Source: CAD feature listing. Evaluate the final solid. Frame: model axes, mm. A direction names the side the tool comes from. Round coordinates to 2 decimals unless told otherwise and drop trailing zeros. Write each loop counter-clockwise with the first axis right and the second up, starting at its lowest first coordinate (ties: lowest second). Pieces come first, ordered by that corner, then holes. Notation, with made-up numbers: (8, 58.5) -> (17, 58.5) arc R16 ccw to (17, 70.5) -> close; hole circle Ø1 at (-8, -17). An arc over 180 degrees is marked (long way). Return JSON: item names as keys, results as strings. Group by question number.
Autodesk Fusion 360 part; units mm, degrees
sketch "Sketch1" plane through (0, 0, 0) normal (0, 0, 1) x (1, 0, 0)
  circle A0 centre (0, 0) radius 12
  dimension "d1" = 24
extrude "Extrude1" add sketch "Sketch1" along normal blind 16.75 makes body 1
sketch "Sketch2" plane through (0, 0, 0) normal (0, 0, 1) x (1, 0, 0)
  circle A0 centre (0, 0) radius 19.75
  dimension "d4" = 39.5
extrude "Extrude2" add sketch "Sketch2" against normal blind 13 bodies 1
sketch "Sketch3" plane through (0, 0, 0) normal (0, 1, 0) x (1, 0, 0)
  line L0 (0, 0) -> (0, -4.94)
  dimension "d7" = 4.94
sketch "Sketch4" plane through (0, 0, 16.75) normal (0, 0, 1) x (-1, 0, 0)
  circle A0 centre (0, 0) radius 12
sketch "Sketch5" plane through (0, 0, 0) normal (0, 1, 0) x (1, 0, 0)
sketch "Sketch6" plane through (0, 0, 0) normal (0, 0, 1) x (1, 0, 0)
  circle A0 centre (0, 0) radius 16
  dimension "d9" = 32
extrude "Extrude3" add sketch "Sketch6" along normal blind 3 separate body makes body 2
move_body "Move1" bodies 2 to x (1, 0, 0) y (0, 1, 0) z (0, 0, 1) at (0, 0, 4.94)
sketch "Sketch7" plane through (0, 0, 7.94) normal (0, 0, 1) x (-1, 0, 0)
  circle A0 centre (0, 0) radius 16
  line L0 (0, 0) -> (13, 16)
  line L1 (0, -2.5) -> (0, -20)
  line L2 (0, 0) -> (-13, 16)
  line L3 (-20, 0) -> (-2.5, 0)
  line L4 (0, 0) -> (13, -16)
  line L5 (0, 0) -> (-13, -16)
  line L6 (-13, 16) -> (-22, 6)
  line L7 (-22, 6) -> (-13, -16)
  line L8 (13, 16) -> (27, 0)
  line L9 (27, 0) -> (13, -16)
extrude "Extrude4" cut sketch "Sketch7" against normal blind 4 contours A0 L0 L4 | A0 L0 L4 L8 L9 | A0 L2 L5 | A0 L2 L3 L6 L7 | A0 L3 L5 L7 bodies 2
sketch "Sketch8" plane through (0, 0, 16.75) normal (0, 0, 1) x (-1, 0, 0)
  circle A0 centre (0, 0) radius 7
  dimension "d14" = 14
extrude "Extrude5" cut sketch "Sketch8" against normal blind 33 bodies 1 2 makes body 3 at (-4.4893, -12.169, 7.94)
combine "Combine1" operation add target body 1 tool bodies 2 3
Item 1: Material intervals for probe 1 along Z at (x, y) = (7, 10); probe 2 along Y at (x, z) = (0, 10); probe 3 along Y at (x, z) = (0, -10.25), sorted ascending.
Item 2: Pull-direction query (Z, two-part tool) for faces 5 (the flat face through (8.81, -10.84, 6.46)), 6 (the cylindrical face through (-11.99, -0.53, 8.26)), 7 (the flat face through (0, 13, 7.94)); classes: +Z half, -Z half, draft (parallel to the pull), parting line (faces both ways), or undercut.
Item 3: Cut plane C-C on z = 6.5. Output: boundary loops of the cut face in (x, y).
Item 4: Cut plane D-D on y = -15. Output: boundary loops of the cut face in (x, z).
Item 5: First-contact query: pin 1 Ø1.5 at (x, z) = (8, -3) entering from +Y; pin 2 Ø8 at (y, z) = (0, 11) entering from -X; pin 3 Ø3 at (x, z) = (-9.5, 9.5) entering from -Y. Flat tips, straight axial feed; report the tip coordinate or a pass-through.
Item 6: Cut plane A-A on x = 0. Output: boundary loops of the cut face in (y, z).
Item 7: Cut plane B-B on y = -3. Output: boundary loops of the cut face in (x, z), and give its area (3 significant figures).
Item 8: Set-up query: faces 1 (the flat face through (0, -13, 4.94)), 2 (the flat face through (0, 13, 4.94)), 3 (the cylindrical face through (0, -16, 6)), 4 (the flat face through (-8.81, 10.84, 6.46)). Return all of +Z, -Z, +X, -X, +Y, -Y with unobstructed straight access to the full face (end or side cutting, diameter ignored); none if empty.
Here are the results:
{
 "1": {"probe 1": "z = -13 to 0, 4.94 to 7.94", "probe 2": "y = -12 to -7, 7 to 12", "probe 3": "y = -19.75 to -7, 7 to 19.75"},
 "2": {"face 5": "draft", "face 6": "undercut", "face 7": "+Z half"},
 "3": {"outline": "(-10.09, -12.42) arc R16 ccw to (10.09, -12.42) -> (7.57, -9.31) arc R12 ccw to (7.57, 9.31) -> (10.09, 12.42) arc R16 ccw to (-10.09, 12.42) -> (-7.57, 9.31) arc R12 ccw to (-7.57, -9.31) -> close; hole circle Ø14 at (0, 0)"},
 "4": {"outline": "(-12.85, -13) -> (12.85, -13) -> (12.85, 0) -> (-12.85, 0) -> close; (-5.57, 4.94) -> (5.57, 4.94) -> (5.57, 7.94) -> (-5.57, 7.94) -> close"},
 "5": {"pin 1": "stops at y = 18.37", "pin 2": "stops at x = -12", "pin 3": "stops at y = -8.94"},
 "6": {"outline": "(-19.75, -13) -> (-7, -13) -> (-7, 16.75) -> (-12, 16.75) -> (-12, 7.94) -> (-16, 7.94) -> (-16, 4.94) -> (-12, 4.94) -> (-12, 0) -> (-19.75, 0) -> close; (7, -13) -> (19.75, -13) -> (19.75, 0) -> (12, 0) -> (12, 4.94) -> (16, 4.94) -> (16, 7.94) -> (12, 7.94) -> (12, 16.75) -> (7, 16.75) -> close"},
 "7": {"outline": "(-19.52, -13) -> (-6.32, -13) -> (-6.32, 16.75) -> (-11.62, 16.75) -> (-11.62, 0) -> (-19.52, 0) -> close; (6.32, -13) -> (19.52, -13) -> (19.52, 0) -> (11.62, 0) -> (11.62, 16.75) -> (6.32, 16.75) -> close", "area": "520 mm^2"},
 "8": {"face 1": "-Y", "face 2": "+Y", "face 3": "+Z, -Y", "face 4": "+Z, -X"}
}
